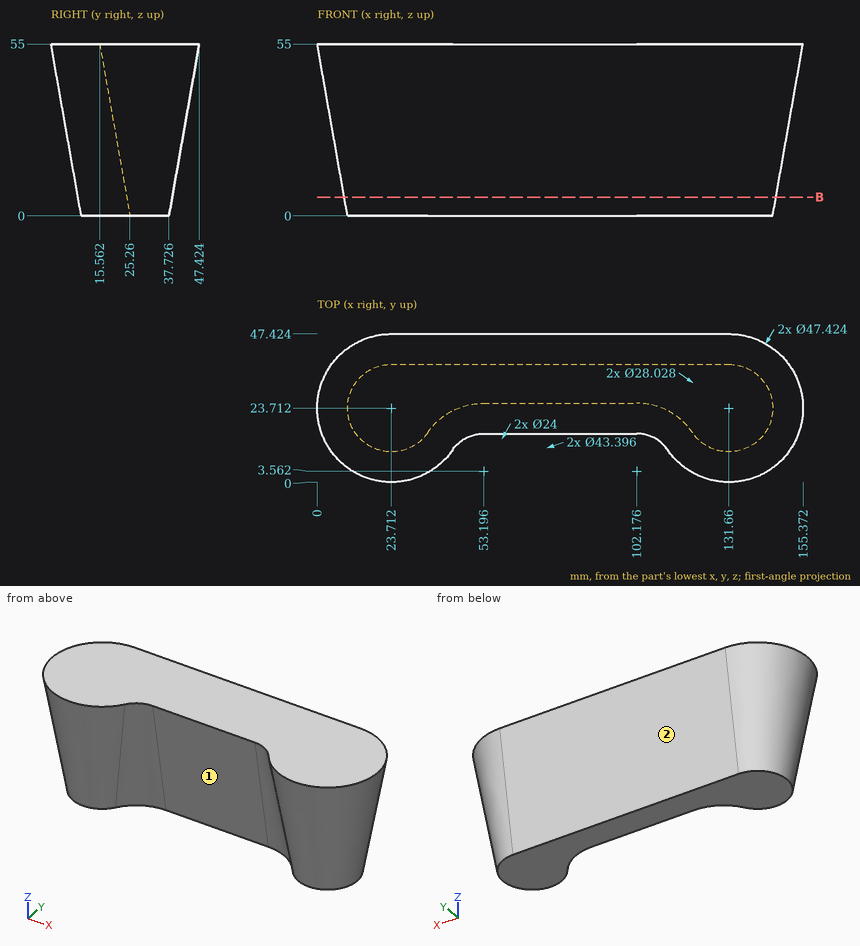
Here's the drawing with two shaded views (mm, measured from the low corner). I have some questions. Coordinates: 2 decimals unless noted, no trailing zeros. Order: outer loops, then holes, each group sorted by start corner. A loop starts at its lowest first (then second) coordinate and runs counter-clockwise, first axis right, second up. Notation, with made-up numbers: (-19, -33) - (9, -33) arc R14 cw to (9, -29) - close; hole circle Ø5 at (-3, 20). An arc over 180 degrees is marked (long way). Use CSV: the item, a comma, the result in double quotes. Start each with the question number.
1. I'm going to push flat-ended pins straight in: pin 1 (5 mm diameter, centred on y = 35.5, z = 21.5, fed in from +X) (1 decimal); pin 2 (6 mm diameter, centred on x = 48.5, z = 15.5, fed in from +Y); pin 3 (6 mm diameter, centred on y = 27.5, z = 16.5, fed in from -X). Where does each tip first touch, or does it pass through?
2. Please list where these lines run through material, in increasing order: line 1 (X direction, y = 12, z = 36) (1 decimal); line 2 (X direction, y = 16, z = 11.5) (1 decimal); line 3 (X direction, y = 23, z = 43) (1 decimal). Write a range as from..to.
3. If we mould it in two halves opening along X, with no side actions, what happens to the marked faces 1 and 2? For each: +X half, -X half, draft (parallel to the pull), parting line (faces both ways), or undercut.
4. Suppose I cut it at B-B on z = 6. List the corners of the cut face in (x, y) for me (1 decimal), then the cut area to 3 significant figures.
Output:
1,pin 1,"stops at x = 146.9"
1,pin 2,"stops at y = 40.99"
1,pin 3,"stops at x = 6.48"
2,line 1,"x = 7.1..40.4, 115..148.3"
2,line 2,"x = 9.6..38, 117.4..145.7"
2,line 3,"x = 2.1..153.2"
3,face 1,"undercut"
3,face 2,"draft"
4,outline,"(23.7, 38.8) arc R15.1 ccw (long way) to (36.2, 15.2) arc R20.6 cw to (53.2, 24.2) - (102.2, 24.2) arc R20.6 cw to (119.2, 15.2) arc R15.1 ccw (long way) to (131.7, 38.8) - close"
4,area,"2,720 mm2"
